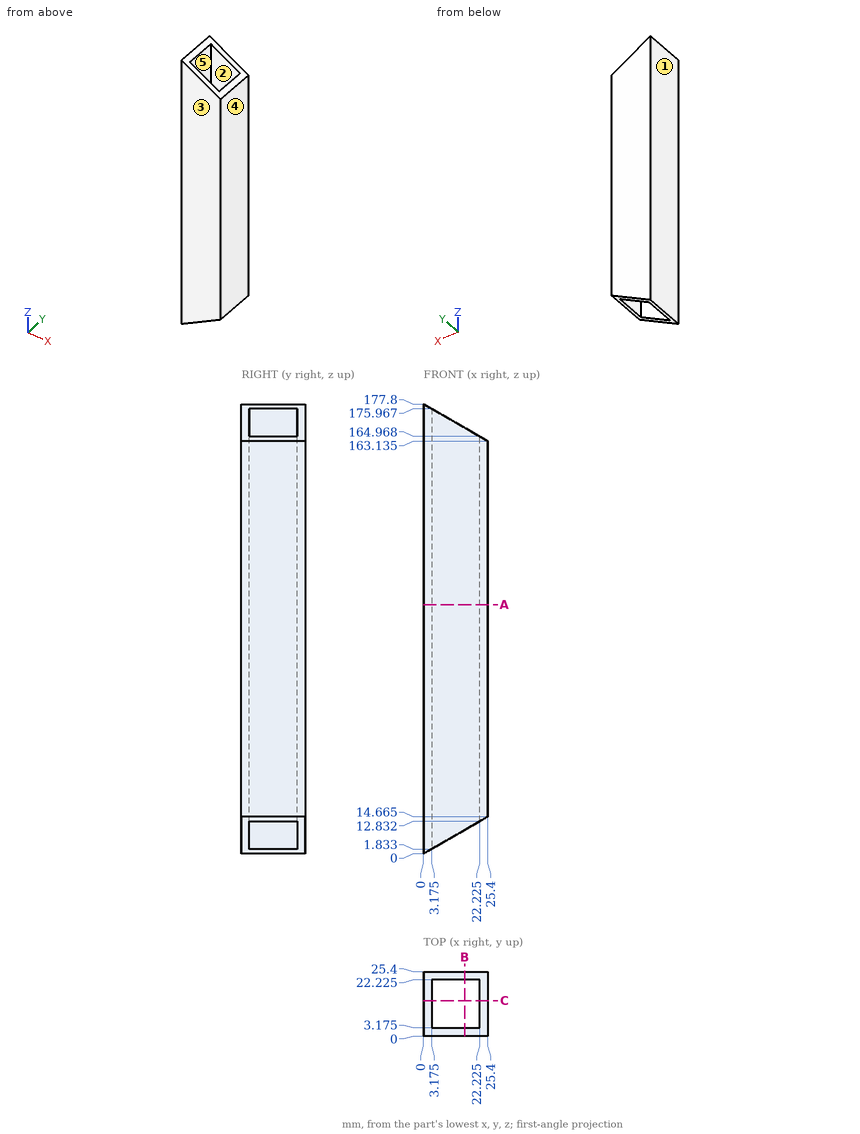
Geometry: see drawing. Coordinates: mm, zero at the bounding-box minimum. A direction names the side the tool comes from. Coordinates: 2 decimals unless noted, no trailing zeros. Loops run counter-clockwise (first coordinate to the right, second up) from the corner with the lowest first, then second, coordinate; pieces in that order, holes last. Notation, with made-up numbers: M 27,51 L 69,51 A26 ccw 69,67 Z; hole C 15.25,23.5 d6. An arc over 180 degrees is marked long. Answer in a Markdown table with one row per item.
1. Section C-C, the plane y = 14. Output: boundary loops of the cut face in (x, z) (1 decimal).
Response:
| item | result |
|---|---|
| outline | M 0,0 L 3.2,1.8 L 3.2,176 L 0,177.8 Z; M 22.2,12.8 L 25.4,14.7 L 25.4,163.1 L 22.2,165 Z |
2. Section A-A, the plane z = 98.5. Output: boundary loops of the cut face in (x, y) (1 decimal).
Response:
| item | result |
|---|---|
| outline | M 0,0 L 25.4,0 L 25.4,25.4 L 0,25.4 Z; hole M 3.2,3.2 L 22.2,3.2 L 22.2,22.2 L 3.2,22.2 Z |
3. Reachability of the marked faces 1 and 2 from +Z, -Z, +X, -X, +Y, -Y: full face, straight path, thin tool, end or side. Return the list, or none.
Response:
| item | result |
|---|---|
| face 1 | +Z, -Z, -X, +Y, -Y |
| face 2 | +Z, -Z |
4. Draft query along Y for the marked faces 3, 4 and 5. Return one class per face: pulls with the +Y half, pulls with the -Y half, needs draft (parallel to the pull), parting line crosses it, or undercut.
Response:
| item | result |
|---|---|
| face 3 | pulls with the -Y half |
| face 4 | needs draft |
| face 5 | undercut |
5. First-contact query: pin 1 (4 mm diameter, centred on x = 6, y = 13, fed in from +Z); pin 2 (3 mm diameter, centred on x = 17.5, y = 4.5, fed in from -Z). Flat tips, straight axial feed; report the tip coordinate or a pass-through.
Response:
| item | result |
|---|---|
| pin 1 | passes through |
| pin 2 | stops at z = 9.7 |
6. Section B-B, the plane x = 16.25. Output: boundary loops of the cut face in (y, z) (1 decimal), then the cut area to 3 significant figures.
Response:
| item | result |
|---|---|
| outline | M 0,9.4 L 3.2,9.4 L 3.2,168.4 L 0,168.4 Z; M 22.2,9.4 L 25.4,9.4 L 25.4,168.4 L 22.2,168.4 Z |
| area | 1,010 mm2 |
7. Material intervals for line 1 (Y direction, x = 5.75, z = 99.5) (1 decimal); line 2 (Z direction, x = 1.75, y = 20.5), sorted ascending.
Response:
| item | result |
|---|---|
| line 1 | y = 0 to 3.2, 22.2 to 25.4 |
| line 2 | z = 1.01 to 176.79 |
